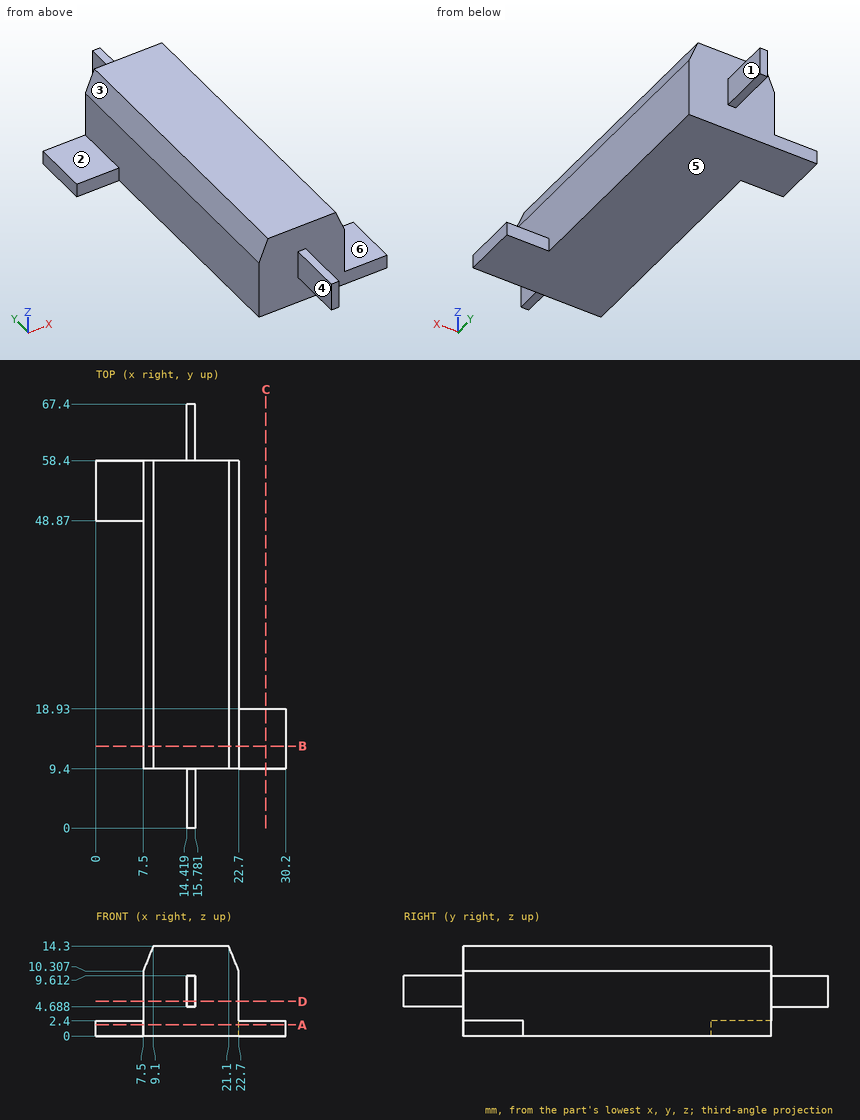
Study the drawing (mm; zero at the part's minimum x, y, z) and answer. A direction names the side the tool comes from. Give positions to 0.01 mm unless a question says otherwise; leave off trailing zeros. Write each loop counter-clockwise with the first axis right and the second up, starting at its lowest first coordinate (ties: lowest second). Pieces come first, ordered by that corner, then holes. Notation, with made-up numbers: (28.5, 49.25) - (80.5, 49.25) arc R27 ccw to (80.5, 65.25) - close; hole circle Ø7 at (36.5, -17.5). An arc over 180 degrees is marked (long way). Use CSV: the item, a comma, the result in double quotes. Start each with the question number.
(1) Find section C-C (x = 27). Give the vertices of the cut face in (y, z).
(2) Given P1, Ø1.1, axis at x = 15, y = 3, coming from the -Z side; P2, Ø8, axis at y = 24.5, z = 7.5, coming from the -X side; P3, Ø4, axis at y = 3.5, z = 6, coming from the -X side; P4, Ø2, axis at x = 25.5, z = 10.5, coming from the +Y side (3 decimals), each flat-ended and moving along its own axis, determine where each tip first touches the part or whether it passes through.
(3) Find section A-A (z = 1.75). Give the vertices of the cut face in (x, y).
(4) Find section D-D (z = 5.5). Give the vertices of the cut face in (x, y), plus the area to 3 significant figures.
(5) For the marked faces 4, 5 and 6, determine the directions among +Z, -Z, +X, -X, +Y, -Y from which every point of the face is accessible in a straight line to the end or side of a thin tool.
(6) Determine the mould class of the marked faces 1, 2 and 3 for opening direction X: +X half, -X half, draft (parallel to the pull), parting line (faces both ways), or undercut.
(7) Find section B-B (y = 13). Give the vertices of the cut face in (x, z), plus the area to 3 significant figures.
(8) Consider line 1 along Z through (x, y) = (2.5, 56.5); line 2 along Y through (x, z) = (11.5, 5.25); line 3 along X through (y, z) = (35, 6.5). Determine where each line is inside the solid, lowest interval first.
Findings below:
1,outline,"(9.4, 0) - (18.93, 0) - (18.93, 2.4) - (9.4, 2.4) - close"
2,P1,"z = 4.69"
2,P2,"x = 7.5"
2,P3,"x = 14.42"
2,P4,"through"
3,outline,"(0, 48.87) - (7.5, 48.87) - (7.5, 9.4) - (30.2, 9.4) - (30.2, 18.93) - (22.7, 18.93) - (22.7, 58.4) - (0, 58.4) - close"
4,outline,"(7.5, 9.4) - (14.42, 9.4) - (14.42, 0) - (15.78, 0) - (15.78, 9.4) - (22.7, 9.4) - (22.7, 58.4) - (15.78, 58.4) - (15.78, 67.4) - (14.42, 67.4) - (14.42, 58.4) - (7.5, 58.4) - close"
4,area,"770 mm2"
5,face 4,"+Z, -Z, -X, -Y"
5,face 5,"-Z, +X, -X, +Y, -Y"
5,face 6,"+Z, +X, +Y, -Y"
6,face 1,"+X half"
6,face 2,"draft"
6,face 3,"-X half"
7,outline,"(7.5, 0) - (30.2, 0) - (30.2, 2.4) - (22.7, 2.4) - (22.7, 10.31) - (21.1, 14.3) - (9.1, 14.3) - (7.5, 10.31) - close"
7,area,"229 mm2"
8,line 1,"0 to 2.4"
8,line 2,"9.4 to 58.4"
8,line 3,"7.5 to 22.7"
